Source: CAD feature listing. Evaluate the final solid. Frame: model axes, mm. Face numbers are marked on the shaded views. Give positions to 0.01 mm unless a question says otherwise; leave off trailing zeros. Loops run counter-clockwise (first coordinate to the right, second up) from the corner with the lowest first, then second, coordinate; pieces in that order, holes last. Notation, with made-up numbers: M -29,21.5 L 16,21.5 A22 ccw 16,50.5 Z; hole C -36,80.25 d1. An arc over 180 degrees is marked long. Put each result on its own line as item: value.
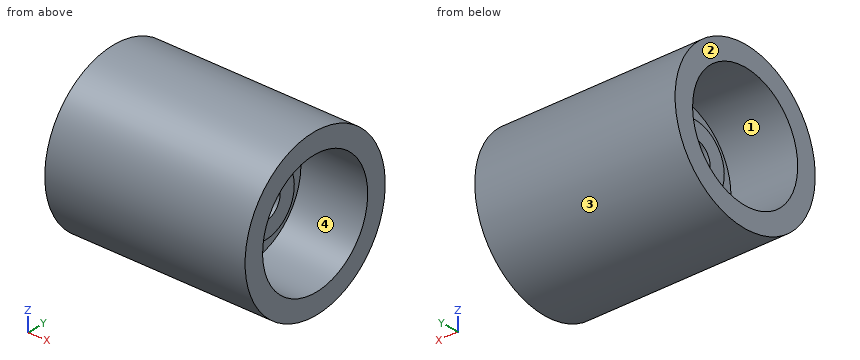
from build123d import *

# Parameters (mm, degrees)
SKETCH2_R          = 2.6
CUT_EXTRUDE1_DEPTH = 29.182441342


with BuildPart() as part:
    # Sketch1 → Revolve1 (revolve)
    with BuildSketch(Plane.XY, mode=Mode.PRIVATE) as revolve1_sk:
        Polygon((-7.5, 0), (-7.5, 5), (-5, 5), (-5, 9), (-15, 9), (-15, 12), (15, 12), (15, 9), (5, 9), (5, 5), (7.5, 5), (7.5, 0), align=None)
    revolve(revolve1_sk.sketch.rotate(Axis((0, 0, 0), (1, 0, 0)), 90), axis=Axis((0, 0, 0), (1, 0, 0)))

    # Sketch2 → Cut-Extrude1 (cut, through all)
    with BuildSketch(Plane.ZY.offset(7.5)):
        Circle(SKETCH2_R)
    extrude(amount=-CUT_EXTRUDE1_DEPTH, mode=Mode.SUBTRACT)


solid = part.part
1. Material intervals for line 1 (Y direction, x = -7, z = 0); line 2 (Y direction, x = -1.5, z = 0); line 3 (X direction, y = 5, z = 5.5), sorted ascending. Write a range as from..to.
Found:
line 1: -12..-9, -5..-2.6, 2.6..5, 9..12
line 2: -12..-2.6, 2.6..12
line 3: -5..5
2. Section query A-A (z = 0). Output: boundary loops of the cut face in (x, y), plus the area to 3 significant figures.
Found:
outline: M -15,-12 L 15,-12 L 15,-9 L 5,-9 L 5,-5 L 7.5,-5 L 7.5,-2.6 L -7.5,-2.6 L -7.5,-5 L -5,-5 L -5,-9 L -15,-9 Z; M -15,9 L -5,9 L -5,5 L -7.5,5 L -7.5,2.6 L 7.5,2.6 L 7.5,5 L 5,5 L 5,9 L 15,9 L 15,12 L -15,12 Z
area: 332 mm^2
3. Contact query for flat-ended pins moving along their axis: P1, Ø9, axis at y = -4, z = -1, coming from the -X side; P2, Ø5, axis at y = 0, z = -2, coming from the +X side; P3, Ø2, axis at y = 1, z = 6.5, coming from the -X side. Output: stop coordinate, or through.
Found:
P1: x = -7.5
P2: x = 7.5
P3: x = -5
4. Section query D-D (z = -3). Output: boundary loops of the cut face in (x, y), plus the area to 3 significant figures.
Found:
outline: M -15,-11.62 L 15,-11.62 L 15,-8.49 L 5,-8.49 L 5,-4 L 7.5,-4 L 7.5,4 L 5,4 L 5,8.49 L 15,8.49 L 15,11.62 L -15,11.62 L -15,8.49 L -5,8.49 L -5,4 L -7.5,4 L -7.5,-4 L -5,-4 L -5,-8.49 L -15,-8.49 Z
area: 398 mm^2
5. Draft query along Y for the marked faces 1, 2, 3 and 4. Return one class per face: pulls with the +Y half, pulls with the -Y half, needs draft (parallel to the pull), parting line crosses it, or undercut.
Found:
face 1: undercut
face 2: needs draft
face 3: parting line crosses it
face 4: undercut
6. Section query C-C (y = -8.5). Output: boundary loops of the cut face in (x, z), plus the area to 3 significant figures.
Found:
outline: M -15,-8.47 L 15,-8.47 L 15,-2.96 L 5,-2.96 L 5,2.96 L 15,2.96 L 15,8.47 L -15,8.47 L -15,2.96 L -5,2.96 L -5,-2.96 L -15,-2.96 Z
area: 390 mm^2
